Verification items for this drawing (mm, ordinates from the low corner). A direction names the side the tool comes from. Give positions to 0.01 mm unless a question says otherwise; leave off trailing zeros. Write each loop counter-clockwise with the first axis right and the second up, starting at its lowest first coordinate (ties: lowest second). Pieces come first, ordered by that corner, then holes. Notation, with made-up numbers: (-17, 41.5) -> (24, 41.5) arc R32 cw to (24, 75.5) -> close; hole circle Ø3 at (66, -18.5). An arc over 180 degrees is marked (long way). Write item = value, one per line.
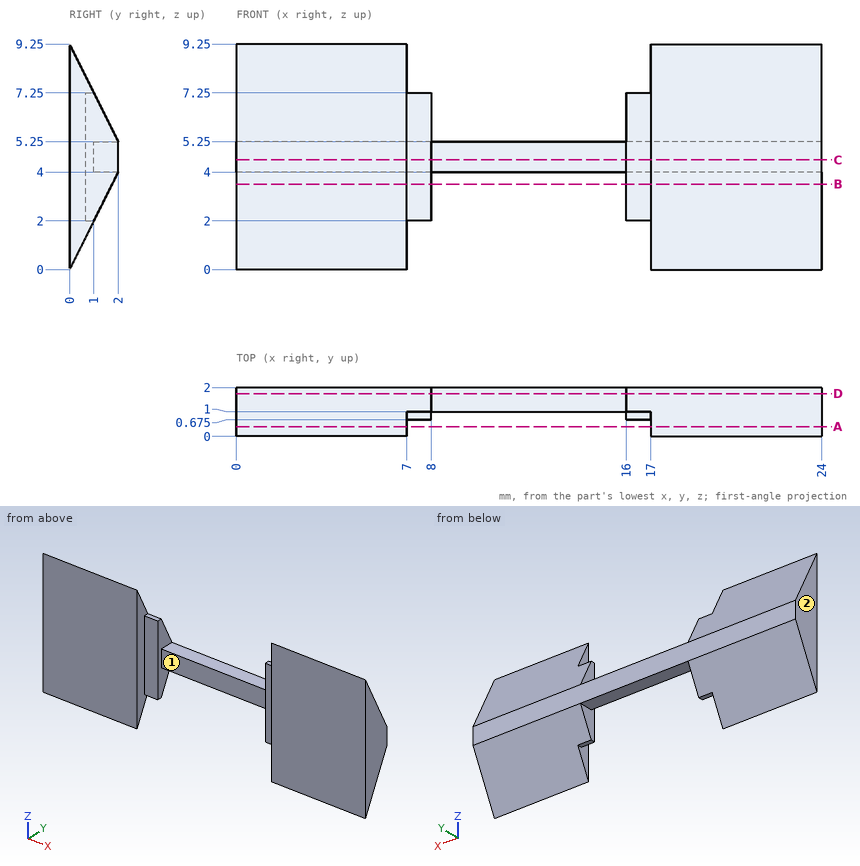
Item 1: Sectioned sample at D-D on y = 1.75. Record the cut outline in (x, z).
Response values:
outline = (0, 3.5) -> (8, 3.5) -> (8, 4) -> (16, 4) -> (16, 3.5) -> (24, 3.5) -> (24, 5.75) -> (16, 5.75) -> (16, 5.25) -> (8, 5.25) -> (8, 5.75) -> (0, 5.75) -> close
Item 2: Sectioned sample at A-A on y = 0.4. Record the cut outline in (x, z).
Response values:
outline = (0, 0.8) -> (7, 0.8) -> (7, 8.45) -> (0, 8.45) -> close; (17, 0.8) -> (24, 0.8) -> (24, 8.45) -> (17, 8.45) -> close
Item 3: Sectioned sample at C-C on z = 4.5. Record the cut outline in (x, y) (3 decimals), then the cut area to 4 significant figures.
Response values:
outline = (0, 0) -> (7, 0) -> (7, 0.675) -> (8, 0.675) -> (8, 1) -> (16, 1) -> (16, 0.675) -> (17, 0.675) -> (17, 0) -> (24, 0) -> (24, 2) -> (0, 2) -> close
area = 38.65 mm^2
Item 4: Go/stop test with flat-tipped pins: P1, Ø3, axis at x = 16, z = 2.5, coming from the -Y side; P2, Ø1.1, axis at x = 13.5, y = 1.5, coming from the +Z side; P3, Ø0.8, axis at x = 7.5, z = 5, coming from the -Y side (3 decimals); P4, Ø1, axis at x = 21.5, y = 2, coming from the +Z side. Record where each tip stops, or that it passes through.
Response values:
P1 = 0
P2 = 5.25
P3 = 0.675
P4 = 6.25
Item 5: Sectioned sample at B-B on z = 3.5. Record the cut outline in (x, y) (3 decimals), then the cut area to 4 significant figures.
Response values:
outline = (0, 0) -> (7, 0) -> (7, 0.675) -> (8, 0.675) -> (8, 1.75) -> (0, 1.75) -> close; (16, 0.675) -> (17, 0.675) -> (17, 0) -> (24, 0) -> (24, 1.75) -> (16, 1.75) -> close
area = 26.65 mm^2
Item 6: Set-up check for the marked faces 1 and 2: record each of +Z, -Z, +X, -X, +Y, -Y from which the full face is reachable in a straight line by a thin tool's end or side.
Response values:
face_1 = +Z, -Z, -Y
face_2 = +Z, -Z, -X, +Y, -Y
Item 7: Material ranges on line 1 (X direction, y = 0.1, z = 2.75); line 2 (X direction, y = 1.2, z = 5.5); line 3 (Z direction, x = 9.25, y = 1.25), recorded low to high.
Response values:
line_1 = 0 to 7, 17 to 24
line_2 = 0 to 8, 16 to 24
line_3 = 4 to 5.25
